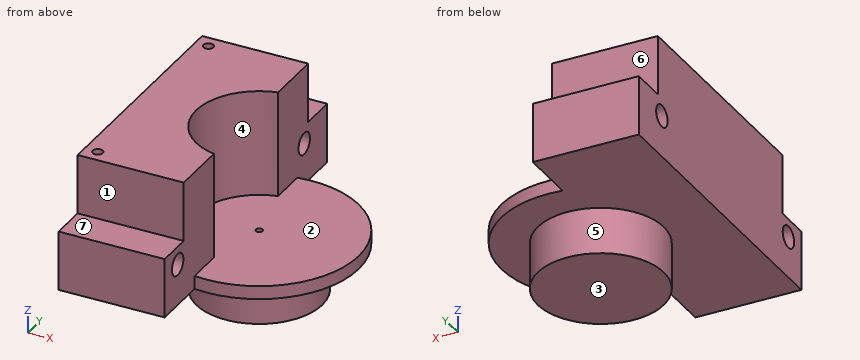
from build123d import *

# Parameters (mm, degrees)
CYLINDER011_R     = 0.5
CYLINDER011_DEPTH = 10
CYLINDER010_R     = 9.5
CYLINDER010_DEPTH = 50
CYLINDER009_R     = 0.75
CYLINDER009_DEPTH = 10
CYLINDER008_R     = 0.75
CYLINDER008_DEPTH = 10
CYLINDER007_R     = 1.65
CYLINDER007_DEPTH = 100
CYLINDER006_R     = 1.65
CYLINDER006_DEPTH = 100
CYLINDER001_R     = 15
CYLINDER001_DEPTH = 2
BOX003_W          = 16
BOX003_H          = 36
BOX003_DEPTH      = 16
BOX004_W          = 16
BOX004_H          = 47
BOX004_DEPTH      = 9
CYLINDER_R        = 9.5
CYLINDER_DEPTH    = 7


with BuildPart() as zylinder011:
    # Cylinder011 → Cylinder011 (new body)
    with BuildSketch(Plane.XY.offset(2)):
        Circle(CYLINDER011_R)
    extrude(amount=CYLINDER011_DEPTH)


with BuildPart() as zylinder010:
    # Cylinder010 → Cylinder010 (new body)
    with BuildSketch(Plane.XY.offset(9)):
        Circle(CYLINDER010_R)
    extrude(amount=CYLINDER010_DEPTH)


with BuildPart() as zylinder009:
    # Cylinder009 → Cylinder009 (new body)
    with BuildSketch(Plane(origin=(-16, -16, 16), x_dir=(1, 0, 0), z_dir=(0, 0, 1))):
        Circle(CYLINDER009_R)
    extrude(amount=CYLINDER009_DEPTH)


with BuildPart() as m1_holes_for_modulation_coil:
    # Cylinder008 → Cylinder008 (new body)
    with BuildSketch(Plane(origin=(-16, 16, 16), x_dir=(1, 0, 0), z_dir=(0, 0, 1))):
        Circle(CYLINDER008_R)
    extrude(amount=CYLINDER008_DEPTH)

    # Compound004: union Zylinder009
    add(zylinder009.part)


with BuildPart() as zylinder007:
    # Cylinder007 → Cylinder007 (new body)
    with BuildSketch(Plane(origin=(-40, -19.75, 13.25), x_dir=(0, 0, -1), z_dir=(1, 0, 0))):
        Circle(CYLINDER007_R)
    extrude(amount=CYLINDER007_DEPTH)


with BuildPart() as compound003:
    # Cylinder006 → Cylinder006 (new body)
    with BuildSketch(Plane(origin=(-40, 16.85, 13.25), x_dir=(0, 0, -1), z_dir=(1, 0, 0))):
        Circle(CYLINDER006_R)
    extrude(amount=CYLINDER006_DEPTH)

    # Compound003: union Zylinder007
    add(zylinder007.part)


with BuildPart() as zylinder001:
    # Cylinder001 → Cylinder001 (new body)
    with BuildSketch(Plane.XY.offset(7)):
        Circle(CYLINDER001_R)
    extrude(amount=CYLINDER001_DEPTH)


with BuildPart() as obj1:
    # Box003 → Box003 (new body)
    with BuildSketch(Plane(origin=(-18, -18, 9), x_dir=(1, 0, 0), z_dir=(0, 0, 1))):
        with Locations((8, 18)):
            Rectangle(BOX003_W, BOX003_H)
    extrude(amount=BOX003_DEPTH)


with BuildPart() as obj2:
    # Box004 → Box004 (new body)
    with BuildSketch(Plane(origin=(-18, -23.5, 7), x_dir=(1, 0, 0), z_dir=(0, 0, 1))):
        with Locations((8, 23.5)):
            Rectangle(BOX004_W, BOX004_H)
    extrude(amount=BOX004_DEPTH)


with BuildPart() as cut005:
    # Cylinder → Cylinder (new body)
    with BuildSketch(Plane.XY):
        Circle(CYLINDER_R)
    extrude(amount=CYLINDER_DEPTH)

    # Fusion: union Zylinder001, obj1, obj2
    add(zylinder001.part)
    add(obj1.part)
    add(obj2.part)

    # Cut002: cut Compound003
    add(compound003.part, mode=Mode.SUBTRACT)

    # Cut003: cut M1 holes for modulation coil
    add(m1_holes_for_modulation_coil.part, mode=Mode.SUBTRACT)

    # Cut004: cut Zylinder010
    add(zylinder010.part, mode=Mode.SUBTRACT)

    # Cut005: cut Zylinder011
    add(zylinder011.part, mode=Mode.SUBTRACT)


solid = cut005.part
Verification items for the finished model (mm, model axes). Face numbers are marked on the shaded views. A direction names the side the tool comes from. Coordinates: 2 decimals unless noted, no trailing zeros. Order: outer loops, then holes, each group sorted by start corner. A loop starts at its lowest first (then second) coordinate and runs counter-clockwise, first axis right, second up. Notation, with made-up numbers: (58.5, 30.5) -> (93.5, 30.5) arc R20 cw to (93.5, 55.5) -> close; hole circle Ø9 at (26.5, -2). An arc over 180 degrees is marked (long way). Use CSV: the item, a comma, the result in double quotes. Start each with the question number.
Q1. Depth check by flat-ended pin: P1, Ø19.5, axis at x = 6, y = -2, coming from the +Z side; P2, Ø1, axis at y = 7, z = 8.5, coming from the +X side; P3, Ø5.5, axis at y = -19.75, z = 13.25, coming from the +X side; P4, Ø2.5, axis at y = 16.85, z = 13.25, coming from the +X side (3 decimals). Enter the tip coordinate at first touch or a pass-through.
Q2. Thickness scan on line 1 along Y through (x, z) = (-10, 13.25); line 2 along Y through (x, z) = (-16, 21.25); line 3 along Y through (x, z) = (-6.5, 13.25). Record the ranges inside material, lowest first.
Q3. Section check A-A, the plane x = -16. Record the cut outline in (y, z).
Q4. Section check C-C, the plane z = 19. Record the cut outline in (x, y), and give its area (3 significant figures).
Q5. Section check D-D, the plane y = -19.75. Record the cut outline in (x, z).
Q6. Section check B-B, the plane z = 13.25. Record the cut outline in (x, y).
Q7. Tool access check on the marked faces 5, 6 and 7. Record the directions out of +Z, -Z, +X, -X, +Y, -Y that give a thin tool (end or side, any length) a straight path to the whole face; none if there is none.
Q8. Draft check along Y on the marked faces 1, 2, 3 and 4. Enter one of: +Y half, -Y half, draft (parallel to the pull), parting line (faces both ways), or undercut.
Returned:
1,P1,"stops at z = 9"
1,P2,"stops at x = 13.52"
1,P3,"stops at x = -2"
1,P4,"passes through"
2,line 1,"y = -23.5 to -21.4, -18.1 to 15.2, 18.5 to 23.5"
2,line 2,"y = -18 to -16.75, -15.25 to 15.25, 16.75 to 18"
2,line 3,"y = -23.5 to -21.4, -18.1 to -6.93, 6.93 to 15.2, 18.5 to 23.5"
3,outline,"(-23.5, 7) -> (23.5, 7) -> (23.5, 16) -> (18, 16) -> (18, 25) -> (16.75, 25) -> (16.75, 16) -> (15.25, 16) -> (15.25, 25) -> (-15.25, 25) -> (-15.25, 16) -> (-16.75, 16) -> (-16.75, 25) -> (-18, 25) -> (-18, 16) -> (-23.5, 16) -> close; hole circle Ø3.3 at (-19.75, 13.25); hole circle Ø3.3 at (16.85, 13.25)"
4,outline,"(-18, -18) -> (-2, -18) -> (-2, -9.29) arc R9.5 cw to (-2, 9.29) -> (-2, 18) -> (-18, 18) -> close; hole circle Ø1.5 at (-16, -16); hole circle Ø1.5 at (-16, 16)"
4,area,"468 mm^2"
5,outline,"(-18, 7) -> (-2, 7) -> (-2, 11.6) -> (-18, 11.6) -> close; (-18, 14.9) -> (-2, 14.9) -> (-2, 16) -> (-18, 16) -> close"
6,outline,"(-18, -23.5) -> (-2, -23.5) -> (-2, -21.4) -> (-18, -21.4) -> close; (-18, -18.1) -> (-2, -18.1) -> (-2, -9.29) arc R9.5 cw to (-2, 9.29) -> (-2, 15.2) -> (-18, 15.2) -> close; (-18, 18.5) -> (-2, 18.5) -> (-2, 23.5) -> (-18, 23.5) -> close"
7,face 5,"-Z"
7,face 6,"+Z, +X, -X, +Y"
7,face 7,"+Z, +X, -X, -Y"
8,face 1,"-Y half"
8,face 2,"undercut"
8,face 3,"draft"
8,face 4,"undercut"
